The model under review builds one solid part; all positions refer to its coordinate system, in mm. A direction names the side the tool comes from. Round coordinates to 2 decimals unless told otherwise and drop trailing zeros. Loops run counter-clockwise (first coordinate to the right, second up) from the corner with the lowest first, then second, coordinate; pieces in that order, holes last. Notation, with made-up numbers: (-17, -15) -> (36, -15) arc R16 cw to (36, 11) -> close; hole circle Ø4 at (-16, 39). An arc over 180 degrees is marked (long way). Write each question's results on one line, items separated by ' | '. Start each with the question number.
Item 1: Tool access review of faces 1 (the cylindrical face through (-7.7, -6.4, 10.1)), 2 (the flat face through (-11, 171.45, 7)), 3 (the cylindrical face through (-2.44, 100.18, 5.89)): name each direction out of +Z, -Z, +X, -X, +Y, -Y from which nothing blocks a thin tool from reaching the whole face with its end or side.
Item 2: We need section B-B (z = 0). Give the boundary of the cut face in (x, y) (3 decimals).
Item 3: We need section D-D (y = 6). Give the boundary of the cut face in (x, z) (3 decimals).
Item 4: We need section C-C (z = 10.5). Give the boundary of the cut face in (x, y), and give its area (3 significant figures).
Item 5: For L1, parallel to X at y = 135, z = 0 (3 decimals); L2, parallel to X at y = -6, z = 0 (3 decimals); L3, parallel to Y at x = -10.5, z = 8, list the stretches that pass through material, from the lowest coordinate up. Write a range as from..to.
Item 6: Clearance check with flat-ended pins moving along their axes: pin 1 Ø1 at (x, y) = (0.5, 64) entering from -Z (3 decimals); pin 2 Ø1 at (x, y) = (-5.5, 139.5) entering from -Z; pin 3 Ø2 at (y, z) = (18.5, -8.5) entering from +X; pin 4 Ø8 at (x, y) = (6, 110) entering from +Z. State where each tip first meets the part, or that it passes through.
Item 7: We need section A-A (x = 0). Give the boundary of the cut face in (y, z) (3 decimals), and give its area (3 significant figures).
Item 8: Mouldability with a two-part tool opening along Z and no side actions: class faces 4 (the flat face through (11, -12.7, 7)), 5 (the flat face through (6, 0, 3)), 6 (the cylindrical face through (7.7, 187.1, 10.1)) as pulls with the +Z half, pulls with the -Z half, needs draft (parallel to the pull), parting line crosses it, or undercut.
from build123d import *

# Parameters (mm, degrees)
SKETCH1_R           = 15.875
SKETCH1_R_2         = 6.3754
BOSS_EXTRUDE1_DEPTH = 203.2
BOSS_EXTRUDE2_START = 12.7
SKETCH2_R           = 15.875
SKETCH2_R_2         = 12.7
BOSS_EXTRUDE2_DEPTH = 12.7
CUT_EXTRUDE1_START  = -31.75
SKETCH3_R           = 15.875
SKETCH3_R_2         = 12.7
CUT_EXTRUDE1_DEPTH  = 31.75


with BuildPart() as part:
    # Sketch1 → Boss-Extrude1 (new body)
    with BuildSketch(Plane(origin=(0, 0, 0), x_dir=(1, 0, 0), z_dir=(0, 1, 0))):
        with Locations(Location((0, 0, 0), (0, 0, 270))):
            Circle(SKETCH1_R)
        with Locations(Location((0, 0, 0), (0, 0, 270))):
            Circle(SKETCH1_R_2, mode=Mode.SUBTRACT)
    extrude(amount=BOSS_EXTRUDE1_DEPTH)

    # Sketch2 → Boss-Extrude2 (add)
    with BuildSketch(Plane.XZ.offset(BOSS_EXTRUDE2_START)):
        with Locations(Location((0, 0, 0), (0, 0, 270))):
            Circle(SKETCH2_R)
        with Locations(Location((0, 0, 0), (0, 0, 270))):
            Circle(SKETCH2_R_2, mode=Mode.SUBTRACT)
    extrude(amount=-BOSS_EXTRUDE2_DEPTH)

    # Sketch3 → Cut-Extrude1 (cut)
    with BuildSketch(Plane(origin=(0, 203.2, 0), x_dir=(1, 0, 0), z_dir=(0, 1, 0)).offset(CUT_EXTRUDE1_START)):
        with Locations(Location((0, 0, 0), (0, 0, 90))):
            Circle(SKETCH3_R)
        with Locations(Location((0, 0, 0), (0, 0, 90))):
            Circle(SKETCH3_R_2, mode=Mode.SUBTRACT)
    extrude(amount=CUT_EXTRUDE1_DEPTH, mode=Mode.SUBTRACT)


solid = part.part
Here are the results:
1) face 1: -Y | face 2: +Y | face 3: +Y, -Y
2) outline: (-15.875, -12.7) -> (-12.7, -12.7) -> (-12.7, 0) -> (-6.375, 0) -> (-6.375, 203.2) -> (-12.7, 203.2) -> (-12.7, 171.45) -> (-15.875, 171.45) -> close; (6.375, 0) -> (12.7, 0) -> (12.7, -12.7) -> (15.875, -12.7) -> (15.875, 171.45) -> (12.7, 171.45) -> (12.7, 203.2) -> (6.375, 203.2) -> close
3) outline: circle Ø31.75 at (0, 0); hole circle Ø12.751 at (0, 0)
4) outline: (-11.91, -12.7) -> (-7.14, -12.7) -> (-7.14, 0) -> (7.14, 0) -> (7.14, -12.7) -> (11.91, -12.7) -> (11.91, 171.45) -> (7.14, 171.45) -> (7.14, 203.2) -> (-7.14, 203.2) -> (-7.14, 171.45) -> (-11.91, 171.45) -> close | area: 4,660 mm2
5) L1: x = -15.875..-6.375, 6.375..15.875 | L2: x = -15.875..-12.7, 12.7..15.875 | L3: y = -12.7..171.45
6) pin 1: stops at z = -15.875 | pin 2: stops at z = -15.07 | pin 3: stops at x = 13.99 | pin 4: stops at z = 15.75
7) outline: (-12.7, -15.875) -> (171.45, -15.875) -> (171.45, -12.7) -> (203.2, -12.7) -> (203.2, -6.375) -> (0, -6.375) -> (0, -12.7) -> (-12.7, -12.7) -> close; (-12.7, 12.7) -> (0, 12.7) -> (0, 6.375) -> (203.2, 6.375) -> (203.2, 12.7) -> (171.45, 12.7) -> (171.45, 15.875) -> (-12.7, 15.875) -> close | area: 3,740 mm2
8) face 4: needs draft | face 5: undercut | face 6: parting line crosses it
